Could you check a few things on this drawing? It's one solid part, dimensions in mm from its lowest x, y, z. Round coordinates to 2 decimals unless told otherwise and drop trailing zeros. Loops run counter-clockwise (first coordinate to the right, second up) from the corner with the lowest first, then second, coordinate; pieces in that order, holes last. Notation, with made-up numbers: M 73.5,84 L 103.5,84 A20 cw 103.5,117 Z; hole C 84.5,30 d9. An arc over 180 degrees is marked long. Return JSON: item names as keys, results as strings.
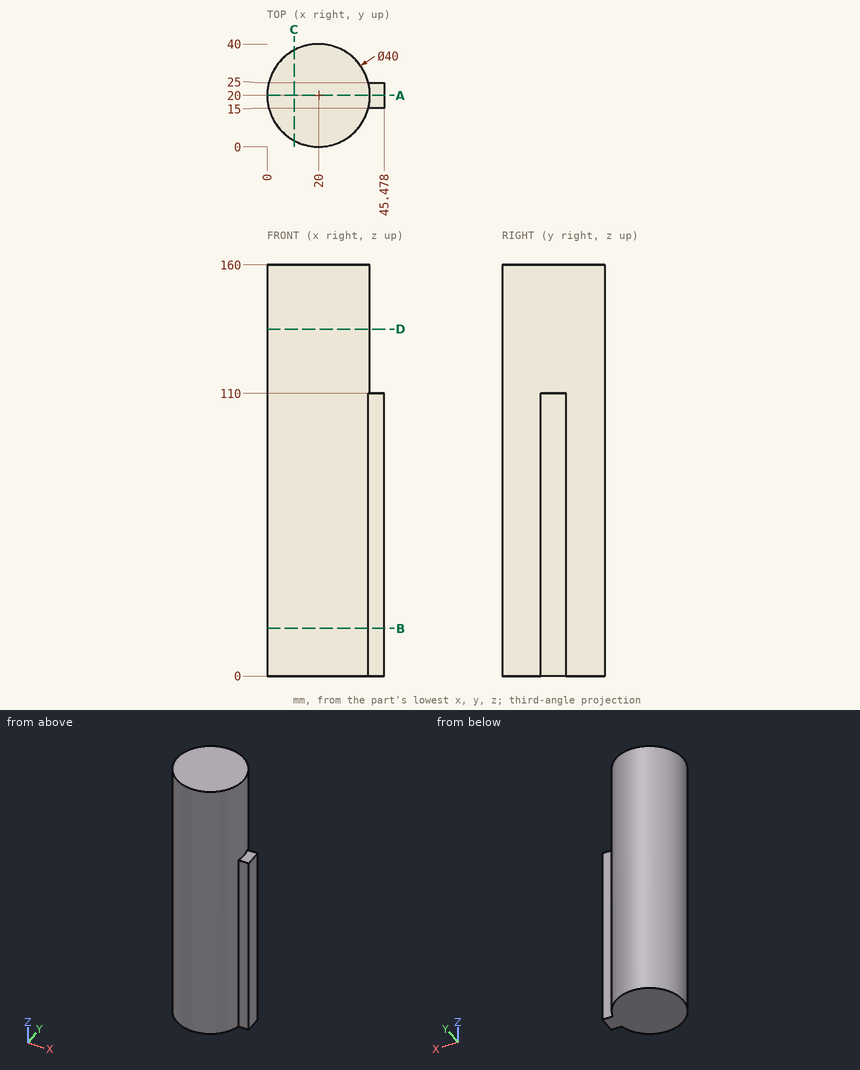
Q1. I'm going to push flat-ended pins straight in: pin 1 Ø3 at (y, z) = (31, 117.5) entering from -X; pin 2 Ø6.5 at (x, z) = (41, 34.5) entering from +Y (1 decimal); pin 3 Ø12 at (x, z) = (7, 65.5) entering from -Y (3 decimals). Where does each tip first touch, or does it pass through?
Results:
{"pin 1": "stops at x = 2.4", "pin 2": "stops at y = 29.2", "pin 3": "stops at y = 1.265"}
Q2. Suppose I cut it at A-A, the plane y = 20. Please give me the cut outline in (x, z), plus the area to 3 significant figures.
Results:
{"outline": "M 0,0 L 45.48,0 L 45.48,110 L 40,110 L 40,160 L 0,160 Z", "area": "7,000 mm2"}
Q3. Suppose I cut it at C-C, the plane x = 10.5. Please give me the cut outline in (y, z), plus the area to 3 significant figures.
Results:
{"outline": "M 2.4,0 L 37.6,0 L 37.6,160 L 2.4,160 Z", "area": "5,630 mm2"}
Q4. Suppose I cut it at B-B, the plane z = 18.5. Please give me the cut outline in (x, y) (1 decimal), plus the area to 3 significant figures.
Results:
{"outline": "M 39.4,15 L 45.5,15 L 45.5,25 L 39.4,25 A20 ccw long Z", "area": "1,310 mm2"}
Q5. If I drill on line 1 along Y through (x, z) = (43, 23); line 2 along Y through (x, z) = (20.5, 150); line 3 along X through (y, z) = (10, 92), over which ranges is the centre line in solid material (lowest first)?
Results:
{"line 1": "y = 15 to 25", "line 2": "y = 0.01 to 39.99", "line 3": "x = 2.68 to 37.32"}
Q6. Suppose I cut it at D-D, the plane z = 135. Please give me the cut outline in (x, y), plus the area to 3 significant figures.
Results:
{"outline": "C 20,20 d40", "area": "1,260 mm2"}
